Can you work these out from the model? Positions are in its coordinate system, mm. A direction names the side the tool comes from. Round coordinates to 2 decimals unless told otherwise and drop trailing zeros. Loops run counter-clockwise (first coordinate to the right, second up) from the corner with the lowest first, then second, coordinate; pieces in that order, holes last. Notation, with made-up numbers: (-8, 73) -> (40, 73) arc R19 ccw to (40, 95) -> close; hole circle Ø4 at (-37.75, -26.75). An arc over 180 degrees is marked (long way). Answer as a JSON object with one key per item and string values.
```python
from build123d import *

# Parameters (mm, degrees)
BOSS_EXTRUDE1_DEPTH = 15.367
SKETCH2_R           = 9.525
BOSS_EXTRUDE2_DEPTH = 7.4168


with BuildPart() as part:
    # Sketch1 → Boss-Extrude1 (new body)
    with BuildSketch(Plane.XY):
        Polygon((7.332348419, 0), (3.666174209, 6.35), (-3.666174209, 6.35), (-7.332348419, 0), (-3.666174209, -6.35), (3.666174209, -6.35), align=None)
        Polygon((5.645908282, 0), (2.822954141, 4.8895), (-2.822954141, 4.8895), (-5.645908282, 0), (-2.822954141, -4.8895), (2.822954141, -4.8895), align=None, mode=Mode.SUBTRACT)
    extrude(amount=BOSS_EXTRUDE1_DEPTH)

    # Sketch2 → Boss-Extrude2 (add)
    with BuildSketch(Plane(origin=(0, 0, 0), x_dir=(-1, 0, 0), z_dir=(0, 0, -1))):
        Circle(SKETCH2_R)
        Polygon((5.645908282, 0), (2.822954141, 4.8895), (-2.822954141, 4.8895), (-5.645908282, 0), (-2.822954141, -4.8895), (2.822954141, -4.8895), align=None, mode=Mode.SUBTRACT)
    extrude(amount=BOSS_EXTRUDE2_DEPTH)


solid = part.part
```
Q1. We'd pull the mould along X, two halves only. Please class faces 1 (the flat face through (0, -6.35, 8)), 2 (the cylindrical face through (7.559, -5.796, -3.656)), 3 (the flat face through (0, 4.89, 4)): pulls with the +X half, pulls with the -X half, needs draft (parallel to the pull), parting line crosses it, or undercut.
Determined:
{"face 1": "needs draft", "face 2": "parting line crosses it", "face 3": "undercut"}
Q2. On a 3-axis mill with a long thin cutter (end or side, diameter ignored), from which of +Z, -Z, +X, -X, +Y, -Y can I reach the whole of each face in a straight line? I mean faces 4 (the flat face through (0, -4.89, 4)), 5 (the flat face through (-6.2, 2.3, 0)), 6 (the flat face through (0, 6.35, 8)). Say none if no direction works.
Determined:
{"face 4": "+Z, -Z", "face 5": "+Z", "face 6": "+Z, +X, -X, +Y"}
Q3. I want a section at D-D, the plane z = 13.25. Write out the boundary of the cut face in (x, y).
Determined:
{"outline": "(-7.33, 0) -> (-3.67, -6.35) -> (3.67, -6.35) -> (7.33, 0) -> (3.67, 6.35) -> (-3.67, 6.35) -> close; hole (-5.65, 0) -> (-2.82, -4.89) -> (2.82, -4.89) -> (5.65, 0) -> (2.82, 4.89) -> (-2.82, 4.89) -> close"}
Q4. I'm going to push flat-ended pins straight in: pin 1 (6 mm diameter, centred on x = -0.5, z = 6, fed in from -Y); pin 2 (8 mm diameter, centred on x = 0, z = 11.5, fed in from +Y); pin 3 (8 mm diameter, centred on y = -6.5, z = 10, fed in from +X); pin 4 (1 mm diameter, centred on y = 7, z = 5.5, fed in from -X). Where does each tip first touch, or does it pass through?
Determined:
{"pin 1": "y = -6.35", "pin 2": "y = 6.35", "pin 3": "x = 5.89", "pin 4": "through"}
Q5. I want a section at C-C, the plane y = -3.25. Write out the boundary of the cut face in (x, z), then the cut area to 3 significant figures.
Determined:
{"outline": "(-8.95, -7.42) -> (-3.77, -7.42) -> (-3.77, 15.37) -> (-5.46, 15.37) -> (-5.46, 0) -> (-8.95, 0) -> close; (3.77, -7.42) -> (8.95, -7.42) -> (8.95, 0) -> (5.46, 0) -> (5.46, 15.37) -> (3.77, 15.37) -> close", "area": "129 mm²"}
Q6. If I drill on L1, parallel to Y at x = 0, z = 13.5; L2, parallel to Z at x = 8.5, y = 0; L3, parallel to Y at x = -2.5, z = -3.75, over which ranges is the centre line in solid material (lowest first)? Write a range as [from, to].
Determined:
{"L1": "[-6.35, -4.89], [4.89, 6.35]", "L2": "[-7.42, 0]", "L3": "[-9.19, -4.89], [4.89, 9.19]"}
